Source: CAD feature listing. Evaluate the final solid. Frame: model axes, mm. A direction names the side the tool comes from. Round coordinates to 2 decimals unless told otherwise and drop trailing zeros. Order: outer loops, then holes, each group sorted by start corner. A loop starts at its lowest first (then second) coordinate and runs counter-clockwise, first axis right, second up. Notation, with made-up numbers: (-39, 19) -> (8, 19) arc R19 cw to (8, 44) -> close; hole circle Ø9 at (-11, 47). An arc over 180 degrees is marked (long way). One line per item, written item: value. Start each with the question number.
1) Mould query, pull axis X, two halves, no side actions, for faces 1 (the face through (-2, -31.75, 10)), 2 (the face through (1.92, -31.01, 9.37)), 3 (the face through (-0.289, -30.945, 10.235)). Classes: pulls with the +X half, pulls with the -X half, needs draft (parallel to the pull), parting line crosses it, or undercut.
2) Section B-B (y = -28). Return the cut outline in (x, z).
3) Section A-A (y = -34). Return the cut outline in (x, z).
4) Ray query, L1, parallel to Z at x = 0.5, y = -33; L2, parallel to X at y = -34.25, z = 5; L3, parallel to Y at x = 6, z = 4.75. Return the intervals inside material, ascending.
5) Reachability of faces 4 (the face through (-2, -30.162, 10)), 5 (the face through (3.34, -26.988, 8.21)) from +Z, -Z, +X, -X, +Y, -Y: full face, straight path, thin tool, end or side. Return the list, or none.
Autodesk Inventor part; units mm, degrees
ref_plane "YZ Plane" through (0, 0, 0) normal (1, 0, 0) x (0, 1, 0)
ref_plane "XZ Plane" through (0, 0, 0) normal (0, 1, 0) x (-1, 0, 0)
ref_plane "XY Plane" through (0, 0, 0) normal (0, 0, 1) x (1, 0, 0)
ref_plane "Work Plane2" through (0.9924, -30.1625, 6.35) normal (-1, 0, 0) x (0, -1, 0)
sketch "Sketch2" plane through (0.9924, -30.1625, 6.35) normal (-1, 0, 0) x (0, -1, 0)
  line L0 (0, -5.5563) -> (0, 3.175)
  line L1 (1.5875, -7.1437) -> (1.5875, 3.175)
  line L2 (0, 7.1741) -> (-1.905, 7.1741)
  line L3 (-3.175, 5.9041) -> (-3.175, 3.2053)
  arc A0 (-1.905, 7.1741) -> (-3.175, 5.9041) centre (-1.905, 5.9041) ccw
  line L4 (12.0631, 0.7938) -> (-37.2001, 0.7938)
  line L5 (-3.175, 3.2053) -> (4.7625, 3.2053)
  line L6 (4.7625, 3.2053) -> (4.7625, 5.9041)
  line L7 (3.4925, 7.1741) -> (1.5875, 7.1741)
  arc A1 (4.7625, 5.9041) -> (3.4925, 7.1741) centre (3.4925, 5.9041) ccw
  line L8 (1.5875, 4.1402) -> (0, 4.1402)
  line L9 (0, 7.1741) -> (0, 4.1402)
  line L10 (1.5875, 7.1741) -> (1.5875, 4.1402)
  point P0 (-30.1625, -6.35)
  point P1 (0, 2.5527)
  point P2 (0, 2.0373)
  point P3 (1.5875, 2.5527)
  dimension "d0" = 1.27
  dimension "d2" = 1.27
  dimension "d4" = 3.9688
  dimension "d5" = 7.9375
revolve "Revolution1" add sketch "Sketch2" angle 360 about axis through (0.9924, -20.447, 7.1438) along (0, 1, 0)
ref_plane "Work Plane3" through (0.9924, -30.9563, 7.1438) normal (0, 0, -1) x (0, -1, 0)
properties part number "Pneumatic_VIAIAR_00090_05"
Findings:
1. face 1: needs draft
1. face 2: undercut
1. face 3: parting line crosses it
2. outline: circle Ø12.71 at (0.99, 7.14); hole circle Ø4.82 at (0.99, 7.14)
3. outline: circle Ø12.67 at (0.99, 7.14); hole circle Ø4.82 at (0.99, 7.14)
4. L1: 0.78 to 4.78, 9.5 to 13.51
4. L2: -4.86 to -0.11, 2.1 to 6.84
4. L3: -34.85 to -31.75, -30.16 to -27.07
5. face 4: none
5. face 5: +Z, -Z, +X, -X, +Y
